Build history of the part. All positions in model axes, mm. Face numbers are marked on the shaded views. A direction names the side the tool comes from. Give positions to 0.01 mm unless a question says otherwise; leave off trailing zeros. Order: outer loops, then holes, each group sorted by start corner. A loop starts at its lowest first (then second) coordinate and runs counter-clockwise, first axis right, second up. Notation, with made-up numbers: (44.5, 59.25) - (82.5, 59.25) arc R28 ccw to (82.5, 83.25) - close; hole circle Ø9 at (56, 24). An arc over 180 degrees is marked (long way). Use a Markdown table: item, result.
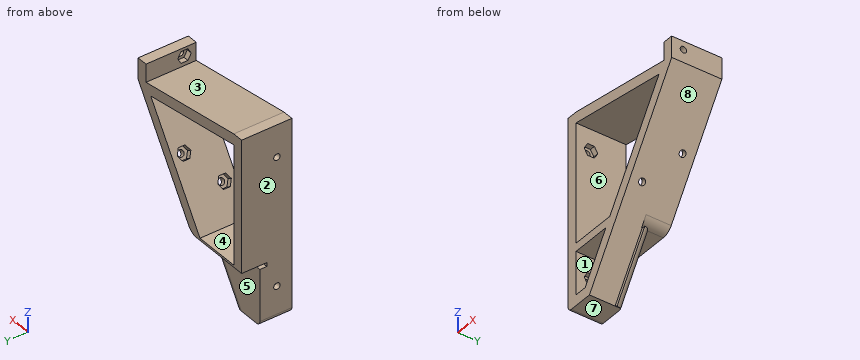
from build123d import *

# Parameters (mm, degrees)
BOSS_EXTRU_1_DEPTH       = 23.5
ESQUISSE10_W             = 28
ESQUISSE10_H             = 8.5
ENL_V_MAT_EXTRU_9_DEPTH  = 114.765108887
ESQUISSE11_W             = 33.386172199
ESQUISSE11_H             = 3
BOSS_EXTRU_2_DEPTH       = 1.5
ESQUISSE12_W             = 1.8
ESQUISSE12_H             = 11.75
ENL_V_MAT_EXTRU_10_DEPTH = 114.765108887
COQUE2_DEPTH             = 23.5
COQUE2_2_DEPTH           = 10.75
COQUE2_START             = 10.75
COQUE2_3_DEPTH           = 3.25
CONG_2_R                 = 2
CONG_3_R                 = 3
ESQUISSE5_R              = 1.5
ENL_V_MAT_EXTRU_4_DEPTH  = 8
ESQUISSE7_R              = 1.5
ENL_V_MAT_EXTRU_6_DEPTH  = 8
ESQUISSE9_R              = 1.5
ENL_V_MAT_EXTRU_8_DEPTH  = 7.5
BOSS_EXTRU_3_DEPTH       = 23.5
BOSS_EXTRU_4_DEPTH       = 10.75
ENL_V_MAT_EXTRU_11_DEPTH = 2.5
ENL_V_MAT_EXTRU_12_DEPTH = 2.5
ENL_V_MAT_EXTRU_13_DEPTH = 2.5
CONG_5_R                 = 6


# Read off the part's stored shape, not the designer's step: Coque2
with BuildPart() as part:
    # Esquisse1 → Boss.-Extru.1 (new body)
    with BuildSketch(Plane(origin=(0, 0, 0), x_dir=(1, 0, 0), z_dir=(0, 1, 0))):
        Polygon((0, 0), (13.5, 0), (65.5, -80.072978118), (65.5, -90), (0, -90), align=None)
    extrude(amount=BOSS_EXTRU_1_DEPTH)

    # Esquisse10 → Enlèv. mat.-Extru.9 (cut, through all)
    with BuildSketch(Plane(origin=(65.5, 0, 0), x_dir=(0, 0, -1), z_dir=(1, 0, 0))):
        with Locations((-14, 19.25)):
            Rectangle(ESQUISSE10_W, ESQUISSE10_H)
    extrude(amount=-ENL_V_MAT_EXTRU_9_DEPTH, mode=Mode.SUBTRACT)

    # Esquisse11 → Boss.-Extru.2 (add)
    with BuildSketch(Plane(origin=(9.495472341, 0, -6.166431839), x_dir=(-0.5446390350150256, 0, -0.838670567945425), z_dir=(0.8386705679454252, 0, -0.5446390350150256))):
        with Locations((-24.045713072, 13.5)):
            Rectangle(ESQUISSE11_W, ESQUISSE11_H)
    extrude(amount=BOSS_EXTRU_2_DEPTH)

    # Esquisse12 → Enlèv. mat.-Extru.10 (cut, through all)
    with BuildSketch(Plane.ZY):
        with Locations((27.1, 17.625)):
            Rectangle(ESQUISSE12_W, ESQUISSE12_H)
    extrude(amount=-ENL_V_MAT_EXTRU_10_DEPTH, mode=Mode.SUBTRACT)

    # Coque2 outline → Coque2 (cut)
    with BuildSketch(Plane(origin=(0, 0, 0), x_dir=(1, 0, 0), z_dir=(0, 1, 0))):
        Polygon((60.5, -81.554045593), (26.371003739, -29), (5, -29), (5, -90), (60.5, -90), align=None)
    extrude(amount=COQUE2_DEPTH, mode=Mode.SUBTRACT)

    # Coque2 2 outline → Coque2 2 (cut)
    with BuildSketch(Plane(origin=(0, 0, 0), x_dir=(1, 0, 0), z_dir=(0, 1, 0))):
        Polygon((10.785221502, -5), (5, -5), (5, -29), (26.371003739, -29), align=None)
    extrude(amount=COQUE2_2_DEPTH, mode=Mode.SUBTRACT)

    # Coque2 3 outline → Coque2 3 (cut)
    with BuildSketch(Plane(origin=(0, 0, 0), x_dir=(1, 0, 0), z_dir=(0, 1, 0)).offset(COQUE2_START)):
        Polygon((23.903254884, -25.2), (10.785221502, -5), (5, -5), (5, -25.2), align=None)
    extrude(amount=COQUE2_3_DEPTH, mode=Mode.SUBTRACT)

    # Congé2
    cong_2_edges = [part.edges().sort_by_distance(p)[0] for p in [
        (0, 7.5, 0),
    ]]
    fillet(cong_2_edges, radius=CONG_2_R)

    # Congé3
    cong_3_edges = [part.edges().sort_by_distance(p)[0] for p in [
        (23.530514866, 15, 12.691520724),
    ]]
    fillet(cong_3_edges, radius=CONG_3_R - 0.0001)  # a hair under: the kernel refuses the full size

    # Esquisse5 → Enlèv. mat.-Extru.4 (cut)
    with BuildSketch(Plane.ZY):
        with Locations((15, 7)):
            Circle(ESQUISSE5_R)
        with Locations((75, 7)):
            Circle(ESQUISSE5_R)
    extrude(amount=-ENL_V_MAT_EXTRU_4_DEPTH, mode=Mode.SUBTRACT)

    # Esquisse7 → Enlèv. mat.-Extru.6 (cut)
    with BuildSketch(Plane(origin=(9.495472341, 0, -6.166431839), x_dir=(-0.5446390350150254, 0, -0.8386705679454252), z_dir=(0.8386705679454252, 0, -0.5446390350150254))):
        with Locations((-54.852626973, 5.5)):
            Circle(ESQUISSE7_R)
        with Locations(Location((-70.828706829, 18, 0), (0, 0, 180))):
            Circle(ESQUISSE7_R)
    extrude(amount=-ENL_V_MAT_EXTRU_6_DEPTH, mode=Mode.SUBTRACT)

    # Esquisse9 → Enlèv. mat.-Extru.8 (cut)
    with BuildSketch(Plane(origin=(65.5, 0, 0), x_dir=(0, 0, -1), z_dir=(1, 0, 0))):
        with Locations((-86, 5.5)):
            Circle(ESQUISSE9_R)
    extrude(amount=-ENL_V_MAT_EXTRU_8_DEPTH, mode=Mode.SUBTRACT)

    # Esquisse13 → Boss.-Extru.3 (add)
    with BuildSketch(Plane.XZ):
        Polygon((60.5, 81.554045593), (5, 90), (5, 84.94243498), (57.510973677, 76.951348682), align=None)
    extrude(amount=-BOSS_EXTRU_3_DEPTH)

    # Esquisse14 → Boss.-Extru.4 (add)
    with BuildSketch(Plane.XZ.offset(-10.75)):
        Polygon((5, 25.2), (23.903254884, 25.2), (26.371003739, 29), (5, 29), align=None)
    extrude(amount=BOSS_EXTRU_4_DEPTH)

    # Esquisse16 → Enlèv. mat.-Extru.11 (cut)
    with BuildSketch(Plane(origin=(5, 0, 0), x_dir=(0, 0, -1), z_dir=(1, 0, 0))):
        Polygon((-72.25, 8.58771324), (-75, 10.175426481), (-77.75, 8.58771324), (-77.75, 5.41228676), (-75, 3.824573519), (-72.25, 5.41228676), align=None)
        Polygon((-12.25, 8.58771324), (-15, 10.175426481), (-17.75, 8.58771324), (-17.75, 5.41228676), (-15, 3.824573519), (-12.25, 5.41228676), align=None)
    extrude(amount=-ENL_V_MAT_EXTRU_11_DEPTH, mode=Mode.SUBTRACT)

    # Esquisse17 → Enlèv. mat.-Extru.12 (cut)
    with BuildSketch(Plane.ZY.offset(-60.5)):
        Polygon((86, 2.324573519), (88.75, 3.91228676), (88.75, 7.08771324), (86, 8.675426481), (83.25, 7.08771324), (83.25, 3.91228676), align=None)
    extrude(amount=-ENL_V_MAT_EXTRU_12_DEPTH, mode=Mode.SUBTRACT)

    # Esquisse18 → Enlèv. mat.-Extru.13 (cut)
    with BuildSketch(Plane(origin=(5.302119501, 0, -3.443236664), x_dir=(0.5446390350150256, 0, 0.838670567945425), z_dir=(-0.8386705679454252, 0, 0.5446390350150256))):
        Polygon((57.602626973, 7.08771324), (54.852626973, 8.675426481), (52.102626973, 7.08771324), (52.102626973, 3.91228676), (54.852626973, 2.324573519), (57.602626973, 3.91228676), align=None)
        Polygon((73.578706829, 19.58771324), (70.828706829, 21.175426481), (68.078706829, 19.58771324), (68.078706829, 16.41228676), (70.828706829, 14.824573519), (73.578706829, 16.41228676), align=None)
    extrude(amount=-ENL_V_MAT_EXTRU_13_DEPTH, mode=Mode.SUBTRACT)

    # Congé5
    cong_5_edges = [part.edges().sort_by_distance(p)[0] for p in [
        (31.68341261, 17.625, 28),
    ]]
    fillet(cong_5_edges, radius=CONG_5_R)


solid = part.part
1) Tool access for the marked faces 5, 6, 7 and 8: list every direction of +Z, -Z, +X, -X, +Y, -Y with a clear straight run to the whole face (end or side of a thin tool).
Computed:
| item | result |
|---|---|
| face 5 | -Z, +X, -X, +Y |
| face 6 | +Y, -Y |
| face 7 | -Z, -X, +Y, -Y |
| face 8 | -Z, +X, -Y |
2) Two-plate mould, pull along Z, no slides. Class the marked faces 1, 2, 3 and 4: +Z half, -Z half, draft (parallel to the pull), parting line (faces both ways), or undercut.
Computed:
| item | result |
|---|---|
| face 1 | undercut |
| face 2 | draft |
| face 3 | +Z half |
| face 4 | undercut |
3) Pin check, flat tips, straight feed: P1, Ø1.2, axis at x = 62, y = 6, coming from the -Z side; P2, Ø12, axis at y = 21, z = 27, coming from the +X side; P3, Ø4, axis at x = 19, y = 4.5, coming from the -Z side; P4, Ø20.5, axis at x = 20, z = 14.5, coming from the -Y side. Stop position of each tip, or through.
Computed:
| item | result |
|---|---|
| P1 | stops at z = 73.76 |
| P2 | stops at x = 34.93 |
| P3 | stops at z = 5.39 |
| P4 | stops at y = 0 |
4) Slice it at A-A (z = 51). Write the cut outline in (x, y).
Computed:
| item | result |
|---|---|
| outline | (0, 0) - (5, 0) - (5, 23.5) - (0, 23.5) - close; (40.66, 0) - (46.62, 0) - (46.62, 23.5) - (40.66, 23.5) - close |
5) Wall check: line 1 (Y direction, x = 64.4, z = 86); line 2 (X direction, y = 5.75, z = 34); line 3 (Z direction, x = 46.5, y = 1.75). Give the ranges that are in metal, low to high. Write a range as from..to.
Computed:
| item | result |
|---|---|
| line 1 | y = 0..4, 7..23.5 |
| line 2 | x = 0..5, 29.62..35.58 |
| line 3 | z = 50.82..60, 78.63..83.68 |
